```python
from build123d import *

# Parameters (mm, degrees)
SKETCH2_R           = 27.5
SKETCH2_R_2         = 4
BOSS_EXTRUDE1_DEPTH = 5


with BuildPart() as part:
    # Sketch1 → Revolve1 (revolve)
    with BuildSketch(Plane(origin=(0, 0, 0), x_dir=(1, 0, 0), z_dir=(0, 1, 0))):
        with BuildLine():
            Line((-200, 27.5), (-150, 27.5))
            ThreePointArc((-150, 27.5), (-144.874368671, 39.874368671), (-132.5, 45))
            Line((-132.5, 45), (132.5, 45))
            ThreePointArc((132.5, 45), (144.874368671, 39.874368671), (150, 27.5))
            Line((150, 27.5), (200, 27.5))
            Line((200, 27.5), (200, 31.5))
            Line((200, 31.5), (153.624630174, 31.5))
            ThreePointArc((153.624630174, 31.5), (146.215866724, 44.05672069), (132.5, 49))
            Line((132.5, 49), (-132.5, 49))
            ThreePointArc((-132.5, 49), (-146.215866724, 44.05672069), (-153.624630174, 31.5))
            Line((-153.624630174, 31.5), (-200, 31.5))
            Line((-200, 31.5), (-200, 27.5))
        make_face()
    revolve(axis=Axis((0, 0, 0), (-1, 0, 0)))

    # Sketch2 → Boss-Extrude1 (add)
    with BuildSketch(Plane.ZY.offset(200)):
        with BuildLine():
            Line((-30, 43.084219849), (-65.357142857, 18.46466565))
            ThreePointArc((-65.357142857, 18.46466565), (-75, 0), (-65.357142857, -18.46466565))
            Line((-65.357142857, -18.46466565), (-30, -43.084219849))
            ThreePointArc((-30, -43.084219849), (0, -52.5), (30, -43.084219849))
            Line((30, -43.084219849), (65.357142857, -18.46466565))
            ThreePointArc((65.357142857, -18.46466565), (75, 0), (65.357142857, 18.46466565))
            Line((65.357142857, 18.46466565), (30, 43.084219849))
            ThreePointArc((30, 43.084219849), (0, 52.5), (-30, 43.084219849))
        make_face()
        Circle(SKETCH2_R, mode=Mode.SUBTRACT)
        with Locations((-52.5, 0)):
            Circle(SKETCH2_R_2, mode=Mode.SUBTRACT)
        with Locations((52.5, 0)):
            Circle(SKETCH2_R_2, mode=Mode.SUBTRACT)
    boss_extrude1 = extrude(amount=BOSS_EXTRUDE1_DEPTH)

    # Mirror1: Boss-Extrude1 across plane
    add(boss_extrude1.mirror(Plane(origin=(0, 0, 0), x_dir=(0, 0, 1), z_dir=(1, 0, 0))))


solid = part.part
```
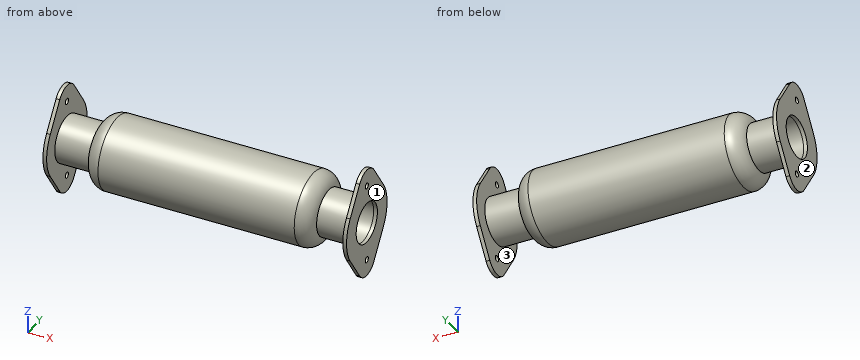
The model under review builds one solid part; all positions refer to its coordinate system, in mm. Face numbers are marked on the shaded views. Round coordinates to 2 decimals unless told otherwise and drop trailing zeros. Write each loop counter-clockwise with the first axis right and the second up, starting at its lowest first coordinate (ties: lowest second). Pieces come first, ordered by that corner, then holes.
(1) Mouldability with a two-part tool opening along X and no side actions: class the marked faces 1, 2 and 3 as +X half, -X half, draft (parallel to the pull), parting line (faces both ways), or undercut.
(2) Insertion check: pin 1 (5 mm diameter, centred on x = 5.5, y = 31.5, fed in from +Z); pin 2 (5 mm diameter, centred on y = 0, z = 52.5, fed in from +X); pin 3 (6 mm diameter, centred on x = 41, z = 16.5, fed in from +Y); pin 4 (3 mm diameter, centred on x = -29.5, y = -39.5, fed in from +Z). Each pin has a flat end and moves straight along its axis. Give the tip position at first contact, or say it passes through.
(3) Wall thickness on L1, parallel to Y at x = -201, z = 0; L2, parallel to X at y = 12.5, z = 50; L3, parallel to Y at x = -202.1, z = -52.5: over which ranges is each line inside the solid? List them lowest first.
(4) We need section C-C on y = 0. Give the number of separate pieces and of enclosed holes in the cut face, and give its area (3 significant figures).
(5) We need section B-B on x = 86.5. Give the boundary of the cut face in (y, z), and give its area (3 significant figures).
Findings below:
1. face 1: +X half
1. face 2: -X half
1. face 3: undercut
2. pin 1: stops at z = 39.5
2. pin 2: passes through
2. pin 3: stops at y = 47.1
2. pin 4: stops at z = 30.94
3. L1: y = -52.5 to -27.5, 27.5 to 52.5
3. L2: x = -205 to -200, 200 to 205
3. L3: y = -27.42 to -4, 4 to 27.42
4. separate pieces: 6
4. enclosed holes: 0
4. area: 4,140 mm2
5. outline: circle Ø98 at (0, 0); hole circle Ø90 at (0, 0)
5. area: 1,180 mm2
